```python
from build123d import *

# Parameters (mm, degrees)
SKETCH2_R           = 2.0828
BOSS_EXTRUDE1_DEPTH = 6.35


with BuildPart() as part:
    # Sketch2 → Boss-Extrude1 (new body)
    with BuildSketch(Plane(origin=(0, 0, 0), x_dir=(1, 0, 0), z_dir=(0, 1, 0))):
        Polygon((63.5, 19.05), (94.930896424, -12.380896424), (90.440768363, -16.871024484), (63.5, -19.05), (50.8, -19.05), (55.245, -6.35), (48.26, 6.35), (21.59, 11.43), (21.59, 19.05), align=None)
        with Locations((58.42, 13.97)):
            Circle(SKETCH2_R, mode=Mode.SUBTRACT)
        with Locations((26.67, 13.97)):
            Circle(SKETCH2_R, mode=Mode.SUBTRACT)
        with Locations((58.42, -13.97)):
            Circle(SKETCH2_R, mode=Mode.SUBTRACT)
    extrude(amount=BOSS_EXTRUDE1_DEPTH)


solid = part.part
```
Can you work these out from the model? Positions are in its coordinate system, mm. A direction names the side the tool comes from. Give positions to 0.01 mm unless a question says otherwise; leave off trailing zeros. Loops run counter-clockwise (first coordinate to the right, second up) from the corner with the lowest first, then second, coordinate; pieces in that order, holes last. Notation, with made-up numbers: M 89.5,-21.75 L 144.5,-21.75 A17 cw 144.5,9.25 Z; hole C 73,88.5 d7. An arc over 180 degrees is marked long. Use CSV: the item, a comma, the result in double quotes. Start each with the question number.
1. Imagine slicing it at B-B, the plane x = 26.67. Write out the boundary of the cut face in (y, z), plus the area to 3 significant figures.
2. For P1, Ø3.5, axis at x = 58.42, z = -13.97, coming from the +Y side; P2, Ø10, axis at x = 50, z = 4.5, coming from the -Y side; P3, Ø1.5, axis at y = 5, z = -1.5, coming from the +X side; P4, Ø1.5, axis at x = 30.5, y = 3, coming from the +Z side, each with a flat end and sliding along its axis, tell me the tip position at first contact or that it passes through.
3. Imagine slicing it at C-C, the plane y = 3.5. Write out the boundary of the cut face in (x, z) (3 decimals).
4. If I drill on L1, parallel to X at y = 3.25, z = -13.97; L2, parallel to Z at x = 58.42, y = 4.5; L3, parallel to Z at x = 27, y = 4, over which ranges is the centre line in solid material (lowest first)?
5. Imagine slicing it at D-D, the plane x = 38. Write out the boundary of the cut face in (y, z), plus the area to 3 significant figures.
6. Imagine slicing it at A-A, the plane z = -13.97. Write out the boundary of the cut face in (x, y), plus the area to 3 significant figures.
7. On a 3-axis mill with a long thin cutter (end or side, diameter ignored), from which of +Z, -Z, +X, -X, +Y, -Y can I reach the whole of each face in a straight line? I mean faces 1 (the face through (59, 6.35, 0)), 2 (the face through (51.8, 3.13, 0.09)). Say none if no direction works.
Response values:
1,outline,"M 0,-19.05 L 6.35,-19.05 L 6.35,-16.05 L 0,-16.05 Z; M 0,-11.89 L 6.35,-11.89 L 6.35,-10.46 L 0,-10.46 Z"
1,area,"28.1 mm^2"
2,P1,"through"
2,P2,"y = 0"
2,P3,"x = 81.8"
2,P4,"z = -9.59"
3,outline,"M 21.59,-19.05 L 63.5,-19.05 L 94.931,12.381 L 90.441,16.871 L 63.5,19.05 L 50.8,19.05 L 55.245,6.35 L 48.26,-6.35 L 21.59,-11.43 Z; hole C 26.67,-13.97 d4.166; hole C 58.42,-13.97 d4.166; hole C 58.42,13.97 d4.166"
4,L1,"21.59 to 24.59, 28.75 to 56.34, 60.5 to 68.58"
4,L2,"-19.05 to -16.05, -11.89 to 11.89, 16.05 to 19.05"
4,L3,"-19.05 to -16.03, -11.91 to -10.4"
5,outline,"M 0,-19.05 L 6.35,-19.05 L 6.35,-8.3 L 0,-8.3 Z"
5,area,"68.2 mm^2"
6,outline,"M 21.59,0 L 24.59,0 L 24.59,6.35 L 21.59,6.35 Z; M 28.75,0 L 56.34,0 L 56.34,6.35 L 28.75,6.35 Z; M 60.5,0 L 68.58,0 L 68.58,6.35 L 60.5,6.35 Z"
6,area,"245 mm^2"
7,face 1,"+Z, -Z, +X, -X, +Y"
7,face 2,"-X, +Y, -Y"
